Build history of the part. All positions in model axes, mm. A direction names the side the tool comes from. Coordinates: 2 decimals unless noted, no trailing zeros. Order: outer loops, then holes, each group sorted by start corner. A loop starts at its lowest first (then second) coordinate and runs counter-clockwise, first axis right, second up. Notation, with made-up numbers: (5, 69.25) - (33, 69.25) arc R22 ccw to (33, 95.25) - close; hole circle Ø6 at (53, 29). An arc over 180 degrees is marked (long way). Write each question's results on one line, items separated by ' | '.
from build123d import *

# Parameters (mm, degrees)
F0_R     = 1
F1_DEPTH = 3.5
F3_DEPTH = 5.5
F4_W     = 11.5
F4_H     = 6.5
F5_DEPTH = 3.5


with BuildPart() as f1:
    # F0 (on Top) → F1 (new body)
    with BuildSketch(Plane.XY):
        Polygon((11.25, -19.485572), (22.5, 0), (11.25, 19.485572), (-11.25, 19.485572), (-22.5, 0), (-11.25, -19.485572), align=None)
        with Locations((-1.5, 0)):
            Circle(F0_R, mode=Mode.SUBTRACT)
        with Locations((1.5, 0)):
            Circle(F0_R, mode=Mode.SUBTRACT)
    extrude(amount=F1_DEPTH)

    # F2 (on face) → F3 (join)
    with BuildSketch(Plane.XY.offset(3.5)):
        Polygon((7.5, 12.990381), (15, 0), (7.5, -12.990381), (-7.5, -12.990381), (-15, 0), (-7.5, 12.990381), (-3.5, 12.990381), (-3.5, 19.485572), (-11.25, 19.485572), (-22.5, 0), (-11.25, -19.485572), (11.25, -19.485572), (22.5, 0), (11.25, 19.485572), (3.5, 19.485572), (3.5, 12.990381), align=None)
    extrude(amount=F3_DEPTH)

    # F4 (on face) → F5 (cut, through all)
    with BuildSketch(Plane.XY.offset(3.5)):
        with Locations((0, 8.5)):
            Rectangle(F4_W, F4_H)
    extrude(amount=-F5_DEPTH, mode=Mode.SUBTRACT)


solid = f1.part
1. Band-saw the part on B-B on z = 1.25. Give the cut face in (x, y).
Solved:
outline: (-22.5, 0) - (-11.25, -19.49) - (11.25, -19.49) - (22.5, 0) - (11.25, 19.49) - (-11.25, 19.49) - close; hole (-5.75, 5.25) - (5.75, 5.25) - (5.75, 11.75) - (-5.75, 11.75) - close; hole circle Ø2 at (-1.5, 0); hole circle Ø2 at (1.5, 0)
2. Probe line 1 (Y direction, x = -1.5, z = 1.4); line 2 (Y direction, x = 6, z = 4.5); line 3 (X direction, y = 0, z = 4.75). List the from-to ranges inside material, lowest first.
Solved:
line 1: y = -19.49 to -1, 1 to 5.25, 11.75 to 19.49 | line 2: y = -19.49 to -12.99, 12.99 to 19.49 | line 3: x = -22.5 to -15, 15 to 22.5
3. Tool access for faces 1 (the face through (3.5, 16, 6)), 2 (the face through (-16.95, -9.61, 4.44)), 3 (the face through (0, 0, 0)), 4 (the face through (0, -12.99, 6)), 5 (the face through (0, 11.75, 2)): list every direction of +Z, -Z, +X, -X, +Y, -Y with a clear straight run to the whole face (end or side of a thin tool).
Solved:
face 1: +Z, +Y | face 2: +Z, -Z, -X, -Y | face 3: -Z, +X, -X, +Y, -Y | face 4: +Z | face 5: +Z, -Z
4. Band-saw the part on D-D on z = 4. Give the cut face in (x, y), then the cut area to 3 significant figures.
Solved:
outline: (-22.5, 0) - (-11.25, -19.49) - (11.25, -19.49) - (22.5, 0) - (11.25, 19.49) - (3.5, 19.49) - (3.5, 12.99) - (7.5, 12.99) - (15, 0) - (7.5, -12.99) - (-7.5, -12.99) - (-15, 0) - (-7.5, 12.99) - (-3.5, 12.99) - (-3.5, 19.49) - (-11.25, 19.49) - close | area: 685 mm2
5. Two-plate mould, pull along X, no slides. Class faces 6 (the face through (16.796, -9.879, 4.437)), 7 (the face through (-6, 12.99, 6)), 8 (the face through (4.7, 13.3, 9)): +X half, -X half, draft (parallel to the pull), parting line (faces both ways), or undercut.
Solved:
face 6: +X half | face 7: undercut | face 8: draft
6. Drop flat-ended pins along their axis: pin 1 Ø1 at (y, z) = (-14.5, 2.5) entering from +X; pin 2 Ø1 at (y, z) = (8, 2.5) entering from -X; pin 3 Ø2 at (y, z) = (13.5, 2) entering from +X. Give the stop position or say it passes through.
Solved:
pin 1: stops at x = 14.42 | pin 2: stops at x = -18.17 | pin 3: stops at x = 15.28
7. Band-saw the part on A-A on x = -1.5. Give the cut face in (y, z), then the cut area to 3 significant figures.
Solved:
outline: (-19.49, 0) - (-1, 0) - (-1, 3.5) - (-12.99, 3.5) - (-12.99, 9) - (-19.49, 9) - close; (1, 0) - (5.25, 0) - (5.25, 3.5) - (1, 3.5) - close; (11.75, 0) - (19.49, 0) - (19.49, 3.5) - (11.75, 3.5) - close | area: 142 mm2
8. Band-saw the part on C-C on y = 8. Give the cut face in (x, z).
Solved:
outline: (-17.88, 0) - (-5.75, 0) - (-5.75, 3.5) - (-10.38, 3.5) - (-10.38, 9) - (-17.88, 9) - close; (5.75, 0) - (17.88, 0) - (17.88, 9) - (10.38, 9) - (10.38, 3.5) - (5.75, 3.5) - close
